The model under review builds one solid part; all positions refer to its coordinate system, in mm. Face numbers are marked on the shaded views. A direction names the side the tool comes from. Coordinates: 2 decimals unless noted, no trailing zeros. Write each loop counter-clockwise with the first axis right and the second up, starting at its lowest first coordinate (ties: lowest second). Pieces come first, ordered by that corner, then holes. Notation, with made-up numbers: (22, -39) - (70, -39) arc R17 ccw to (70, -15) - close; hole circle Ø8 at (-22.75, 31.5). An arc over 180 degrees is marked (long way). Return JSON: item names as keys, results as strings. Group by question number.
(1) Draft analysis for pull direction Z (two halves, no side actions). For the marked faces 1, 2 and 3, state which applies: released by +Z, released by -Z, zero draft, split by the parting line, or undercut.
(2) We need section D-D on x = 74.5. State the section outline as (y, z) points (3 decimals), then the cut area to 3 significant figures.
(3) We need section B-B on y = -58. State the section outline as (x, z) points.
(4) For pin 1 Ø1.5 at (x, z) = (41.5, 55.5) entering from -Y; pin 2 Ø17.5 at (y, z) = (-28.5, 80) entering from +X; pin 3 Ø2.5 at (x, y) = (86, -2.5) entering from -Z (3 decimals); pin 4 Ø12.5 at (x, z) = (77.85, 44.45) entering from +Y, all flat-tipped, find the tip position at first contact; note any pin that passes through.
(5) To check wall thickness, follow L1, parallel to X at y = -1, z = 44; L2, parallel to Z at x = 28, y = -33.5; L3, parallel to Y at x = 65, z = 62. State the ranges of each line that lie inside material, in increasing order. Write a range as from..to.
(6) We need section A-A on x = 25.4. Give the number of separate pieces and of enclosed holes in the cut face, then the cut area to 3 significant figures.
(7) Tool access review of the marked faces 4, 5, 6, 7 and 8: name each direction out of +Z, -Z, +X, -X, +Y, -Y from which nothing blocks a thin tool from reaching the whole face with its end or side.
(8) We need section C-C on y = -50.5. State the section outline as (x, z) points.
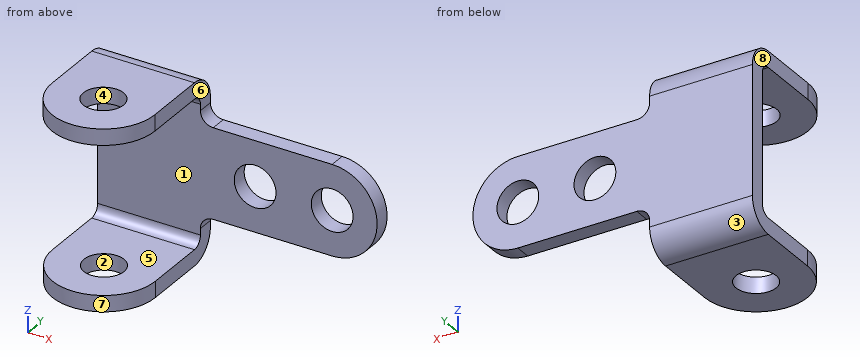
```python
from build123d import *

# Parameters (mm, degrees)
F0_R     = 10.3251
F1_DEPTH = 7.9629
F2_R     = 9.92251
F3_DEPTH = 7.9375
F4_R     = 9.92251
F5_DEPTH = 7.9629
F6_R     = 12.7
F7_R     = 4.7625


with BuildPart() as f1:
    # F0 (on Front) → F1 (new body)
    with BuildSketch(Plane.XZ):
        with BuildLine():
            Line((0, 88.9), (0, 0))
            Line((0, 0), (50.8, 0))
            Line((50.8, 0), (50.8, 15.875))
            ThreePointArc((50.8, 15.875), (52.6598719395, 20.3651280605), (57.15, 22.225))
            Line((57.15, 22.225), (65.1503875852, 22.225))
            Line((65.1503875852, 22.225), (115.9503875852, 22.225))
            ThreePointArc((115.9503875852, 22.225), (138.1753875852, 44.45), (115.9503875852, 66.675))
            Line((115.9503875852, 66.675), (65.1503875852, 66.675))
            Line((65.1503875852, 66.675), (57.15, 66.675))
            ThreePointArc((57.15, 66.675), (52.6598719395, 68.5348719395), (50.8, 73.025))
            Line((50.8, 73.025), (50.8, 88.9))
            Line((50.8, 88.9), (0, 88.9))
        make_face()
        with Locations((77.8503875852, 44.45)):
            Circle(F0_R, mode=Mode.SUBTRACT)
        with Locations((115.9503875852, 44.45)):
            Circle(F0_R, mode=Mode.SUBTRACT)
    extrude(amount=F1_DEPTH)

    # F2 (on Top) → F3 (join)
    with BuildSketch(Plane.XY):
        with BuildLine():
            Line((0, 0), (0, -44.0251193941))
            ThreePointArc((0, -44.0251193941), (25.4, -69.4251193941), (50.8, -44.0251193941))
            Line((50.8, -44.0251193941), (50.8, 0))
            Line((50.8, 0), (0, 0))
        make_face()
        with Locations((25.4, -44.0251193941)):
            Circle(F2_R, mode=Mode.SUBTRACT)
    extrude(amount=F3_DEPTH)

    # F4 (on face) → F5 (join)
    with BuildSketch(Plane.XY.offset(88.9)):
        with BuildLine():
            Line((50.8, -44.45), (50.8, -7.9629))
            Line((50.8, -7.9629), (0, -7.9629))
            Line((0, -7.9629), (0, -44.45))
            ThreePointArc((0, -44.45), (25.4, -69.85), (50.8, -44.45))
        make_face()
        with Locations((25.4, -44.45)):
            Circle(F4_R, mode=Mode.SUBTRACT)
    extrude(amount=-F5_DEPTH)

    # F6
    f6_edges = [f1.edges().sort_by_distance(p)[0] for p in [
        (25.4, 0, 0),
        (25.4, 0, 88.9),
    ]]
    fillet(f6_edges, radius=F6_R)

    # F7
    f7_edges = [f1.edges().sort_by_distance(p)[0] for p in [
        (25.4, -7.9629, 7.9375),
        (25.4, -7.9629, 80.9371),
    ]]
    fillet(f7_edges, radius=F7_R)


solid = f1.part
```
Ans:
{
 "1": {"face 1": "undercut", "face 2": "zero draft", "face 3": "released by -Z"},
 "2": {"outline": "(-7.963, 22.225) - (0, 22.225) - (0, 34.684) - (-7.963, 34.684) - close; (-7.963, 54.216) - (0, 54.216) - (0, 66.675) - (-7.963, 66.675) - close", "area": "198 mm²"},
 "3": {"outline": "(3.92, 80.94) - (46.88, 80.94) - (46.88, 88.9) - (3.92, 88.9) - close; (4.19, 0) - (46.61, 0) - (46.61, 7.94) - (4.19, 7.94) - close"},
 "4": {"pin 1": "y = -7.96", "pin 2": "x = 50.8", "pin 3": "z = 22.225", "pin 4": "through"},
 "5": {"L1": "0..67.54, 88.17..105.64, 126.27..138.17", "L2": "0..7.94, 80.94..88.9", "L3": "-7.96..0"},
 "6": {"separate pieces": "3", "enclosed holes": "0", "area": "1,310 mm²"},
 "7": {"face 4": "+Z", "face 5": "+X, -X, -Y", "face 6": "+Z, +X, +Y, -Y", "face 7": "-Z, -Y", "face 8": "+Z, -Z, -X, +Y, -Y"},
 "8": {"outline": "(0.73, 80.94) - (17.54, 80.94) - (17.54, 88.9) - (0.73, 88.9) - close; (0.84, 0) - (17.88, 0) - (17.88, 7.94) - (0.84, 7.94) - close; (32.92, 0) - (49.96, 0) - (49.96, 7.94) - (32.92, 7.94) - close; (33.26, 80.94) - (50.07, 80.94) - (50.07, 88.9) - (33.26, 88.9) - close"}
}
